```python
from build123d import *

# Parameters (mm, degrees)
F1_DEPTH = 14.224
F2_DEPTH = 7.874
F3_DEPTH = 7.874
F5_DEPTH = 4.826
F6_DEPTH = 25.4
F7_W     = 4.826
F7_H     = 28.575
F8_DEPTH = 6.35


with BuildPart() as f1:
    # F0 (on Front) → F1 (new body, symmetric)
    with BuildSketch(Plane.XZ):
        Polygon((-44.3352609873, 15.875), (-44.3352609873, 0), (-44.3352609873, -15.875), (25.2607390127, -15.875), (25.2607390127, 0), (25.2607390127, 15.875), align=None)
    extrude(amount=F1_DEPTH, both=True)

    # F0 (on Front) → F2 (join, symmetric)
    with BuildSketch(Plane.XZ):
        Polygon((25.2607390127, -15.875), (-44.3352609873, -15.875), (-44.3352609873, -44.45), (60.3127390127, -44.45), (31.7377390127, -15.875), align=None)
        with BuildLine():
            ThreePointArc((9.7667390127, -24.638), (13.718051706, -26.2746873067), (15.3547390127, -30.226))
            ThreePointArc((15.3547390127, -30.226), (13.7180517062, -34.177312693), (9.7667390134, -35.814))
            Line((9.7667390134, -35.814), (-14.1092609873, -35.814))
            ThreePointArc((-14.1092609873, -35.814), (-18.0605736806, -34.1773126933), (-19.6972609873, -30.226))
            ThreePointArc((-19.6972609873, -30.226), (-18.0605736745, -26.2746873007), (-14.1092609702, -24.638))
            Line((-14.1092609702, -24.638), (9.7667390127, -24.638))
        make_face(mode=Mode.SUBTRACT)
    extrude(amount=F2_DEPTH, both=True)

    # F0 (on Front) → F3 (join, symmetric)
    with BuildSketch(Plane.XZ):
        Polygon((-44.3352609873, 44.45), (-44.3352609873, 15.875), (25.2607390127, 15.875), (31.7377390127, 15.875), (60.3127390127, 44.45), align=None)
        with BuildLine():
            ThreePointArc((-19.6972609873, 30.226), (-18.0605736806, 34.1773126933), (-14.1092609873, 35.814))
            Line((-14.1092609873, 35.814), (9.7667390127, 35.814))
            ThreePointArc((9.7667390127, 35.814), (13.718051706, 34.1773126933), (15.3547390127, 30.226))
            ThreePointArc((15.3547390127, 30.226), (13.718051706, 26.2746873067), (9.7667390127, 24.638))
            Line((9.7667390127, 24.638), (-14.1092610119, 24.638))
            ThreePointArc((-14.1092610119, 24.638), (-18.0605736893, 26.2746873154), (-19.6972609873, 30.226))
        make_face(mode=Mode.SUBTRACT)
    extrude(amount=F3_DEPTH, both=True)

    # F4 (on face) → F5 (join)
    with BuildSketch(Plane.XZ.offset(7.874)):
        Polygon((60.3127390127, 44.45), (25.2607390127, 44.45), (25.2607390127, 26.924), (42.7867390127, 26.924), align=None)
        Polygon((25.2607390127, -44.45), (60.3127390127, -44.45), (42.7867390127, -26.924), (25.2607390127, -26.924), align=None)
    extrude(amount=F5_DEPTH)

    # F6 (add): faces of the model
    f6_faces = [f1.faces().sort_by_distance(p)[0] for p in [
        (38.8920723461, -12.7, 36.6606666667),
        (38.8920723461, -12.7, -36.6606666667),
    ]]
    extrude(f6_faces, amount=-F6_DEPTH)

    # F7 (on face) → F8 (cut)
    with BuildSketch(Plane(origin=(-44.3352609873, 0, 0), x_dir=(0, -1, 0), z_dir=(-1, 0, 0))):
        with Locations((5.461, 30.1625)):
            Rectangle(F7_W, F7_H)
        with Locations((5.461, -30.1625)):
            Rectangle(F7_W, F7_H)
    extrude(amount=-F8_DEPTH, mode=Mode.SUBTRACT)


solid = f1.part
```
Verification items for the finished model (mm, model axes). A direction names the side the tool comes from. Round coordinates to 2 decimals unless told otherwise and drop trailing zeros. Order: outer loops, then holes, each group sorted by start corner. A loop starts at its lowest first (then second) coordinate and runs counter-clockwise, first axis right, second up.
1) Cross-section at D-D, the plane x = 29.5. Record the cut outline in (y, z) (3 decimals), plus the area to 3 significant figures.
Geometry says:
outline: (-12.7, -44.45) - (12.7, -44.45) - (12.7, -26.924) - (7.874, -26.924) - (7.874, -15.875) - (-7.874, -15.875) - (-7.874, -26.924) - (-12.7, -26.924) - close; (-12.7, 26.924) - (-7.874, 26.924) - (-7.874, 15.875) - (7.874, 15.875) - (7.874, 26.924) - (12.7, 26.924) - (12.7, 44.45) - (-12.7, 44.45) - close
area: 1,240 mm2
2) Cross-section at A-A, the plane x = 12. Record the cut outline in (y, z) (3 decimals).
Geometry says:
outline: (-14.224, -15.875) - (-7.874, -15.875) - (-7.874, -25.104) - (7.874, -25.104) - (7.874, -15.875) - (14.224, -15.875) - (14.224, 15.875) - (7.874, 15.875) - (7.874, 25.104) - (-7.874, 25.104) - (-7.874, 15.875) - (-14.224, 15.875) - close; (-7.874, -44.45) - (7.874, -44.45) - (7.874, -35.348) - (-7.874, -35.348) - close; (-7.874, 35.348) - (7.874, 35.348) - (7.874, 44.45) - (-7.874, 44.45) - close
3) Cross-section at B-B, the plane z = -28.5. Record the cut outline in (x, y).
Geometry says:
outline: (-44.34, -3.05) - (-37.99, -3.05) - (-37.99, -7.87) - (-19.42, -7.87) - (-19.42, 7.87) - (-44.34, 7.87) - close; (15.08, -7.87) - (25.26, -7.87) - (25.26, -12.7) - (44.36, -12.7) - (44.36, 12.7) - (25.26, 12.7) - (25.26, 7.87) - (15.08, 7.87) - close
4) Draft check along X on faces 5 (the flat face through (25.261, 0, 0)), 6 (the flat face through (-2, 0, -24.638)), 7 (the flat face through (-11, 7.874, -24)), 8 (the flat face through (25.261, -10, 36)). Enter one of: +X half, -X half, draft (parallel to the pull), parting line (faces both ways), or undercut.
Geometry says:
face 5: +X half
face 6: undercut
face 7: draft
face 8: -X half
5) Material ranges on line 1 (Z direction, x = -9, y = 7.5); line 2 (Z direction, x = 25.5, y = -12.5); line 3 (Y direction, x = 21, z = 38.5), recorded low to high.
Geometry says:
line 1: z = -44.45 to -35.81, -24.64 to 24.64, 35.81 to 44.45
line 2: z = -44.45 to -26.92, 26.92 to 44.45
line 3: y = -7.87 to 7.87
6) Cross-section at C-C, the plane y = 4.75. Record the cut outline in (x, z) (3 decimals), plus the area to 3 significant figures.
Geometry says:
outline: (-44.335, -44.45) - (60.313, -44.45) - (31.738, -15.875) - (25.261, -15.875) - (25.261, 15.875) - (31.738, 15.875) - (60.313, 44.45) - (-44.335, 44.45) - close; hole (-14.109, -35.814) - (9.767, -35.814) arc R5.588 ccw to (9.767, -24.638) - (-14.109, -24.638) arc R5.588 ccw to start; hole (-14.109, 24.638) - (9.767, 24.638) arc R5.588 ccw to (9.767, 35.814) - (-14.109, 35.814) arc R5.588 ccw to start
area: 6,640 mm2
7) Tool access check on faces 1 (the flat face through (34, -10, -26.924)), 2 (the flat face through (34, 10, -26.924)), 3 (the flat face through (25.261, -10, -36)), 4 (the flat face through (28, 0, 15.875)). Record the directions out of +Z, -Z, +X, -X, +Y, -Y that give a thin tool (end or side, any length) a straight path to the whole face; none if there is none.
Geometry says:
face 1: +X, -X, -Y
face 2: +X, -X, +Y
face 3: -Z, -X, -Y
face 4: +X, +Y, -Y
8) Depth check by flat-ended pin: pin 1 (4 mm diameter, centred on y = 4, z = -6, fed in from +X); pin 2 (1 mm diameter, centred on x = 13.5, z = 35, fed in from -Y); pin 3 (3.5 mm diameter, centred on x = -16.5, y = -8, fed in from -Z); pin 4 (1.9 mm diameter, centred on x = -2, y = 12.5, fed in from -Z) (3 decimals). Enter the tip coordinate at first touch or a pass-through.
Geometry says:
pin 1: stops at x = 25.26
pin 2: stops at y = -7.87
pin 3: stops at z = -44.45
pin 4: stops at z = -15.875
